Geometry: final body of the model. Coordinates: model frame, mm. Face numbers are marked on the shaded views. A direction names the side the tool comes from. Round coordinates to 2 decimals unless told otherwise and drop trailing zeros. Order: outer loops, then holes, each group sorted by start corner. A loop starts at its lowest first (then second) coordinate and runs counter-clockwise, first axis right, second up. Notation, with made-up numbers: M 86.25,7.25 L 116.25,7.25 A21 ccw 116.25,13.25 Z; hole C -20,20 d3. An arc over 180 degrees is marked long. Put each result on its own line as item: value. Start each with the question number.
1) First-contact query: P1, Ø6, axis at x = -8.5, z = -5, coming from the +Y side; P2, Ø5, axis at y = -31.5, z = -3.5, coming from the -X side; P3, Ø1, axis at y = -33.5, z = 10.5, coming from the -X side. Flat tips, straight axial feed; report the tip coordinate or a pass-through.
2) Draft query along X for the marked faces 1, 2 and 3. Return one class per face: pulls with the +X half, pulls with the -X half, needs draft (parallel to the pull), parting line crosses it, or undercut.
3) Section C-C, the plane y = -30.5. Return loops of the section in (x, z).
4) Section A-A, the plane z = 0. Return loops of the section in (x, y).
5) Access query for the marked faces 4 and 5. Directions: +Z, -Z, +X, -X, +Y, -Y. A direction counts if a zero-diameter tool reaches every point of the face in a straight line with its end or side. Return the directions, or none.
6) Section D-D, the plane z = -17. Return loops of the section in (x, y), then the cut area to 3 significant figures.
7) Section B-B, the plane x = -1. Return loops of the section in (y, z).
8) Material intervals for probe 1 along Z at (x, y) = (0, -16); probe 2 along Z at (x, y) = (0, -28); probe 3 along Y at (x, z) = (18, -7), sorted ascending. Write a range as [from, to].
from build123d import *

# Parameters (mm, degrees)
F0_R     = 17.758511
F0_R_2   = 11.167133
F1_DEPTH = 38.1
F0_W     = 51.393282
F0_H     = 42.341057
F2_DEPTH = 25.4


with BuildPart() as f1:
    # F0 (on Front) → F1 (new body)
    with BuildSketch(Plane.XZ):
        Circle(F0_R)
        Circle(F0_R_2, mode=Mode.SUBTRACT)
    extrude(amount=F1_DEPTH)

    # F0 (on Front) → F2 (join)
    with BuildSketch(Plane.XZ):
        with Locations((-0.438012, 0.292006)):
            Rectangle(F0_W, F0_H)
        Circle(F0_R, mode=Mode.SUBTRACT)
    extrude(amount=F2_DEPTH)


solid = f1.part
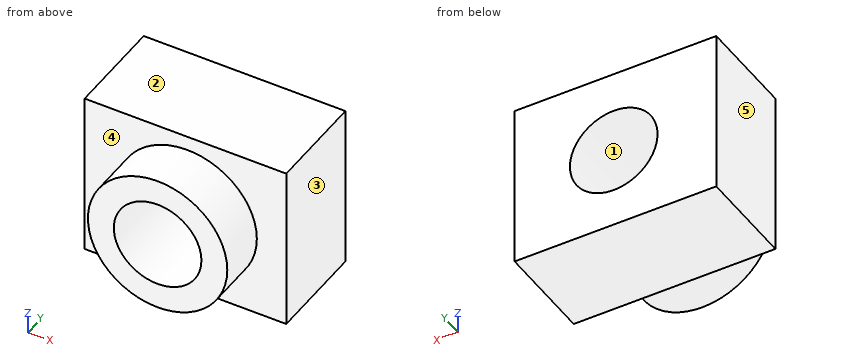
Result sheet:
1. P1: stops at y = 0
1. P2: stops at x = -17.73
1. P3: stops at x = -14.68
2. face 1: undercut
2. face 2: needs draft
2. face 3: pulls with the +X half
3. outline: C 0,0 d35.52; hole C 0,0 d22.33
4. outline: M -26.13,-25.4 L -17.76,-25.4 L -17.76,-38.1 L -11.17,-38.1 L -11.17,0 L -26.13,0 Z; M 11.17,-38.1 L 17.76,-38.1 L 17.76,-25.4 L 25.26,-25.4 L 25.26,0 L 11.17,0 Z
5. face 4: -Y
5. face 5: +Z, -Z, -X, +Y, -Y
6. outline: M -26.13,-25.4 L -5.13,-25.4 L -5.13,-38.1 L 5.13,-38.1 L 5.13,-25.4 L 25.26,-25.4 L 25.26,0 L -26.13,0 Z
6. area: 1,440 mm2
7. outline: M -38.1,-17.73 L -25.4,-17.73 L -25.4,-20.88 L 0,-20.88 L 0,-11.12 L -38.1,-11.12 Z; M -38.1,11.12 L 0,11.12 L 0,21.46 L -25.4,21.46 L -25.4,17.73 L -38.1,17.73 Z
8. probe 1: z = [-20.88, -11.17], [11.17, 21.46]
8. probe 2: z = [-17.76, -11.17], [11.17, 17.76]
8. probe 3: y = [-25.4, 0]
